Could you check a few things on this model? Use its own coordinates, in mm. A direction names the side the tool comes from. Round coordinates to 2 decimals unless told otherwise and drop trailing zeros. Loops run counter-clockwise (first coordinate to the right, second up) from the corner with the lowest first, then second, coordinate; pieces in that order, holes last. Notation, with made-up numbers: (-28, -37.5) - (-13, -37.5) arc R12 ccw to (-13, -28.5) - close; hole circle Ø7 at (37.25, 66). An arc over 180 degrees is marked (long way). Use one line per item in the form item = value.
```python
from build123d import *

# Parameters (mm, degrees)
F1_DEPTH = 38.1
F2_W     = 120.65
F2_H     = 76.2
F3_DEPTH = 38.101


with BuildPart() as f1:
    # F0 (on Front) → F1 (new body)
    with BuildSketch(Plane.XZ):
        Polygon((98.425, 128.5875), (-98.425, 128.5875), (-98.425, -128.5875), (-76.2, -128.5875), (-76.2, -125.4125), (76.2, -125.4125), (76.2, -128.5875), (98.425, -128.5875), (98.425, -90.4875), (-3.175, -90.4875), (-3.175, -39.6875), (98.425, -39.6875), align=None)
    extrude(amount=F1_DEPTH)

    # F2 (on face) → F3 (cut, through all)
    with BuildSketch(Plane.XZ.offset(38.1)):
        with Locations((0, 68.2625)):
            Rectangle(F2_W, F2_H)
    extrude(amount=-F3_DEPTH, mode=Mode.SUBTRACT)


solid = f1.part
```
1. On a 3-axis mill with a long thin cutter (end or side, diameter ignored), from which of +Z, -Z, +X, -X, +Y, -Y can I reach the whole of each face in a straight line? I mean faces 4 (the face through (-1, -19, -125.412)), 5 (the face through (-1, -19, 30.162)), 6 (the face through (48, -19, -90.488)), 7 (the face through (-1, -38.1, 2)), 8 (the face through (87, -19, -128.588)). Say none if no direction works.
Solution:
face_4 = -Z, +Y, -Y
face_5 = +Y, -Y
face_6 = +X, +Y, -Y
face_7 = +Z, -Z, +X, -X, -Y
face_8 = -Z, +X, -X, +Y, -Y
2. Please list where these lines run through material, in increasing order: line 1 along Z through (x, y) = (18.5, -6.5); line 2 along X through (y, z) = (-35, 71) (3 decimals); line 3 along Z through (x, y) = (-37.5, -34).
Solution:
line_1 = -125.41 to -90.49, -39.69 to 30.16, 106.36 to 128.59
line_2 = -98.425 to -60.325, 60.325 to 98.425
line_3 = -125.41 to 30.16, 106.36 to 128.59
3. For P1, Ø3, axis at x = 16, y = -25, coming from the -Z side, with a flat end and sliding along its axis, tell me the tip position at first contact or that it passes through.
Solution:
P1 = -125.41
4. If we section it at C-C, the plane x = 35: Write out the boundary of the cut face in (y, z).
Solution:
outline = (-38.1, -125.41) - (0, -125.41) - (0, -90.49) - (-38.1, -90.49) - close; (-38.1, -39.69) - (0, -39.69) - (0, 30.16) - (-38.1, 30.16) - close; (-38.1, 106.36) - (0, 106.36) - (0, 128.59) - (-38.1, 128.59) - close
5. If we section it at D-D, the plane y = -10: Write out the boundary of the cut face in (x, z) (1 decimal).
Solution:
outline = (-98.4, -128.6) - (-76.2, -128.6) - (-76.2, -125.4) - (76.2, -125.4) - (76.2, -128.6) - (98.4, -128.6) - (98.4, -90.5) - (-3.2, -90.5) - (-3.2, -39.7) - (98.4, -39.7) - (98.4, 128.6) - (-98.4, 128.6) - close; hole (-60.3, 30.2) - (60.3, 30.2) - (60.3, 106.4) - (-60.3, 106.4) - close
6. If we section it at A-A, the plane x = -20.5: Write out the boundary of the cut face in (y, z).
Solution:
outline = (-38.1, -125.41) - (0, -125.41) - (0, 30.16) - (-38.1, 30.16) - close; (-38.1, 106.36) - (0, 106.36) - (0, 128.59) - (-38.1, 128.59) - close
7. If we section it at B-B, the plane z = 95: Write out the boundary of the cut face in (x, y) (3 decimals), plus the area to 3 significant figures.
Solution:
outline = (-98.425, -38.1) - (-60.325, -38.1) - (-60.325, 0) - (-98.425, 0) - close; (60.325, -38.1) - (98.425, -38.1) - (98.425, 0) - (60.325, 0) - close
area = 2,900 mm^2
8. We'd pull the mould along X, two halves only. Please class faces 1 (the face through (-60.325, -19, 68)), 2 (the face through (98.425, -19, 43)), 3 (the face through (-87, -19, -128.588)): +X half, -X half, draft (parallel to the pull), parting line (faces both ways), or undercut.
Solution:
face_1 = undercut
face_2 = +X half
face_3 = draft
